```python
from build123d import *

# Parameters (mm, degrees)
CYLINDER940_R          = 6.5
CYLINDER940_DEPTH      = 1
CYLINDER940_ROLL_ANGLE = 90
BOX536_W               = 40.6
BOX536_H               = 38
BOX536_DEPTH           = 20
CYLINDER864_R          = 2.8
CYLINDER864_DEPTH      = 10
CYLINDER864_ROLL_ANGLE = 90
BOX537_W               = 53.4
BOX537_H               = 4
BOX537_DEPTH           = 20


with BuildPart() as cylinder1083:
    # Cylinder940 → Cylinder940 (new body)
    with BuildSketch(Plane.XY):
        Circle(CYLINDER940_R)
    extrude(amount=CYLINDER940_DEPTH)


with BuildPart() as cylinder1083_1:
    # Cylinder940 roll: moved
    add(cylinder1083.part.rotate(Axis((0, 0, 0), (1, 0, 0)), CYLINDER940_ROLL_ANGLE))


with BuildPart() as cylinder1083_2:
    # Cylinder940 placement: moved
    add(cylinder1083_1.part.moved(Location((37, 66.5, -11))))


with BuildPart() as cube:
    # Box536 → Box536 (new body)
    with BuildSketch(Plane(origin=(-0.3, 0, 0), x_dir=(1, 0, 0), z_dir=(0, 0, 1))):
        with Locations((20.3, 19)):
            Rectangle(BOX536_W, BOX536_H)
    extrude(amount=BOX536_DEPTH)


with BuildPart() as cylinder1026:
    # Cylinder864 → Cylinder864 (new body)
    with BuildSketch(Plane.XY):
        Circle(CYLINDER864_R)
    extrude(amount=CYLINDER864_DEPTH)


with BuildPart() as cylinder1026_1:
    # Cylinder864 roll: moved
    add(cylinder1026.part.rotate(Axis((0, 0, 0), (1, 0, 0)), CYLINDER864_ROLL_ANGLE))


with BuildPart() as cylinder1026_2:
    # Cylinder864 placement: moved
    add(cylinder1026_1.part.moved(Location((10, 5, 10))))


with BuildPart() as steering_servo:
    # Box537 → Box537 (new body)
    with BuildSketch(Plane(origin=(-6.7, 7, 0), x_dir=(1, 0, 0), z_dir=(0, 0, 1))):
        with Locations((26.7, 2)):
            Rectangle(BOX537_W, BOX537_H)
    extrude(amount=BOX537_DEPTH)

    # Fusion585: union Cube, Cylinder1026
    add(cube.part)
    add(cylinder1026_2.part)


with BuildPart() as steering_servo_1:
    # Fusion585 placement: moved
    add(steering_servo.part.moved(Location((27, 66.5, -21))))

    # Fusion588: union Cylinder1083
    add(cylinder1083_2.part)


with BuildPart() as steering_servo_2:
    # Fusion588 placement: moved
    add(steering_servo_1.part.moved(Location((1, 0, 0))))


solid = steering_servo_2.part
```
Check sheet for the modelled part. Datum: model origin and axes. Units: mm. A direction names the side the tool comes from. Coordinates: 2 decimals unless noted, no trailing zeros. Order: outer loops, then holes, each group sorted by start corner. A loop starts at its lowest first (then second) coordinate and runs counter-clockwise, first axis right, second up. Notation, with made-up numbers: (69.25, 61) -> (103.25, 61) arc R22 cw to (103.25, 92) -> close; hole circle Ø4 at (-4.75, 3). An arc over 180 degrees is marked (long way). Write item = value, one per line. Start each with the question number.
1) Material ranges on L1, parallel to Y at x = 30.5, z = -15.25; L2, parallel to X at y = 69, z = -6; L3, parallel to Y at x = 34.5, z = -14.75, recorded low to high.
2) Cross-section at C-C (y = 72). Enter the section's corners in (x, z).
3) Go/stop test with flat-tipped pins: P1, Ø10, axis at y = 95.5, z = -15, coming from the -X side; P2, Ø5, axis at x = 72, z = -12.5, coming from the -Y side; P3, Ø3.5, axis at y = 69.5, z = -15.5, coming from the +X side. Record where each tip stops, or that it passes through.
4) Access from +Z, -Z, +X, -X, +Y, -Y to the whole of each face (thin tool, end or side, straight path). Record for faces 1 (the cylindrical face through (31.506, 66.007, -10.714)), 2 (the flat face through (27.7, 70, -11)), 3 (the flat face through (24, 77.5, -11)), 4 (the flat face through (68.3, 70, -11)), 5 (the flat face through (68.3, 91, -11)).
5) Cross-section at D-D (z = -11). Enter the section's corners in (x, y).
6) Cross-section at B-B (z = -16). Enter the section's corners in (x, y).
7) Cross-section at A-A (x = 38). Enter the section's corners in (y, z), then the cut area to 3 significant figures.
Ans:
q1.L1 = 66.5 to 104.5
q1.L2 = 27.7 to 68.3
q1.L3 = 65.5 to 104.5
q2.outline = (27.7, -21) -> (68.3, -21) -> (68.3, -1) -> (27.7, -1) -> close
q3.P1 = 27.7
q3.P2 = 73.5
q3.P3 = 68.3
q4.face_1 = -Y
q4.face_2 = +Z, -Z, -X, -Y
q4.face_3 = +Z, -Z, -X, +Y
q4.face_4 = +Z, -Z, +X, -Y
q4.face_5 = +Z, -Z, +X, +Y
q5.outline = (21.3, 73.5) -> (27.7, 73.5) -> (27.7, 66.5) -> (31.5, 66.5) -> (31.5, 65.5) -> (35.2, 65.5) -> (35.2, 61.5) -> (40.8, 61.5) -> (40.8, 65.5) -> (44.5, 65.5) -> (44.5, 66.5) -> (68.3, 66.5) -> (68.3, 73.5) -> (74.7, 73.5) -> (74.7, 77.5) -> (68.3, 77.5) -> (68.3, 104.5) -> (27.7, 104.5) -> (27.7, 77.5) -> (21.3, 77.5) -> close
q6.outline = (21.3, 73.5) -> (27.7, 73.5) -> (27.7, 66.5) -> (33.85, 66.5) -> (33.85, 65.5) -> (42.15, 65.5) -> (42.15, 66.5) -> (68.3, 66.5) -> (68.3, 73.5) -> (74.7, 73.5) -> (74.7, 77.5) -> (68.3, 77.5) -> (68.3, 104.5) -> (27.7, 104.5) -> (27.7, 77.5) -> (21.3, 77.5) -> close
q7.outline = (61.5, -13.8) -> (65.5, -13.8) -> (65.5, -17.5) -> (66.5, -17.5) -> (66.5, -21) -> (104.5, -21) -> (104.5, -1) -> (66.5, -1) -> (66.5, -4.5) -> (65.5, -4.5) -> (65.5, -8.2) -> (61.5, -8.2) -> close
q7.area = 795 mm²
